Geometry: final body of the model. Coordinates: model frame, mm. Face numbers are marked on the shaded views. A direction names the side the tool comes from. Round coordinates to 2 decimals unless told otherwise and drop trailing zeros. Loops run counter-clockwise (first coordinate to the right, second up) from the corner with the lowest first, then second, coordinate; pieces in that order, holes last. Notation, with made-up numbers: M 52.5,46.25 L 59.5,46.25 A13 cw 59.5,57.25 Z; hole C 59.5,38 d7. An arc over 180 degrees is marked long. Return JSON: item names as keys, results as strings.
from build123d import *

# Parameters (mm, degrees)
PAD003_DEPTH    = 7.5
SKETCH007_W     = 37
SKETCH007_H     = 37
SKETCH007_W_2   = 32.5
SKETCH007_H_2   = 32.5
PAD004_DEPTH    = 66.72
CHAMFER_SIZE    = 2
CHAMFER001_SIZE = 2.9999
POCKET_DEPTH    = 74.421
POCKET001_DEPTH = 18.501


with BuildPart() as part:
    # Sketch006 → Pad003 (new body, symmetric)
    with BuildSketch(Plane.XY):
        Polygon((-16.25, 16.25), (16.25, 16.25), (16.25, -16.25), (6, -16.25), (6, -13.25), (13.25, -13.25), (13.25, 13.25), (-13.25, 13.25), (-13.25, -13.25), (-6, -13.25), (-6, -16.25), (-16.25, -16.25), align=None)
    extrude(amount=PAD003_DEPTH, both=True)

    # Sketch007 (on DatumPlane) → Pad004 (join)
    with BuildSketch(Plane.XY.offset(66.92)):
        Rectangle(SKETCH007_W, SKETCH007_H)
        Rectangle(SKETCH007_W_2, SKETCH007_H_2, mode=Mode.SUBTRACT)
    extrude(amount=-PAD004_DEPTH)

    # Chamfer
    chamfer_edges = [part.edges().sort_by_distance(p)[0] for p in [
        (18.5, -18.5, 33.56),
        (-18.5, -18.5, 33.56),
        (-18.5, 18.5, 33.56),
        (18.5, 18.5, 33.56),
        (-16.25, -16.25, 37.21),
        (16.25, 16.25, 37.21),
        (16.25, -16.25, 37.21),
        (-16.25, 16.25, 37.21),
        (-13.25, 13.25, 0),
        (13.25, 13.25, 0),
        (13.25, -13.25, 0),
        (-13.25, -13.25, 0),
        (16.25, -16.25, -3.65),
        (-16.25, -16.25, -3.65),
        (-16.25, 16.25, -3.65),
        (16.25, 16.25, -3.65),
    ]]
    chamfer(chamfer_edges, length=CHAMFER_SIZE)

    # Chamfer001
    chamfer001_edges = [part.edges().sort_by_distance(p)[0] for p in [
        (-16.25, 0, 7.5),
        (-15.25, 15.25, 7.5),
        (0, 16.25, 7.5),
        (15.25, 15.25, 7.5),
        (16.25, 0, 7.5),
        (15.25, -15.25, 7.5),
        (10.125, -16.25, 7.5),
        (-15.25, -15.25, 7.5),
        (-10.125, -16.25, 7.5),
    ]]
    chamfer(chamfer001_edges, length=CHAMFER001_SIZE)

    # Sketch (on DatumPlane) → Pocket (cut, through all)
    with BuildSketch(Plane.XY.offset(66.92)):
        Polygon((-13.2501, -13.007401), (-13.25, -11.25), (-11.25, -13.25), (-13.007401, -13.2501), align=None)
        Polygon((11.25, -13.25), (13.007401, -13.2501), (13.2501, -13.007401), (13.25, -11.25), align=None)
        Polygon((-13.25, 11.25), (-11.25, 13.25), (-13.007501, 13.25), (-13.2501, 13.007401), align=None)
        Polygon((11.25, 13.25), (13.25, 11.25), (13.2501, 13.007401), (13.007401, 13.2501), align=None)
    extrude(amount=-POCKET_DEPTH, mode=Mode.SUBTRACT)

    # Sketch008 → Pocket001 (cut, through all)
    with BuildSketch(Plane(origin=(0, 0, -17.5), x_dir=(-1, 0, 0), z_dir=(0, -1, 0))):
        with BuildLine():
            Line((-6, -10), (6, -10))
            Line((6, -10), (6, -20))
            ThreePointArc((-6, -20), (0, -26), (6, -20))
            Line((-6, -20), (-6, -10))
        make_face()
    extrude(amount=POCKET001_DEPTH, mode=Mode.SUBTRACT)


solid = part.part
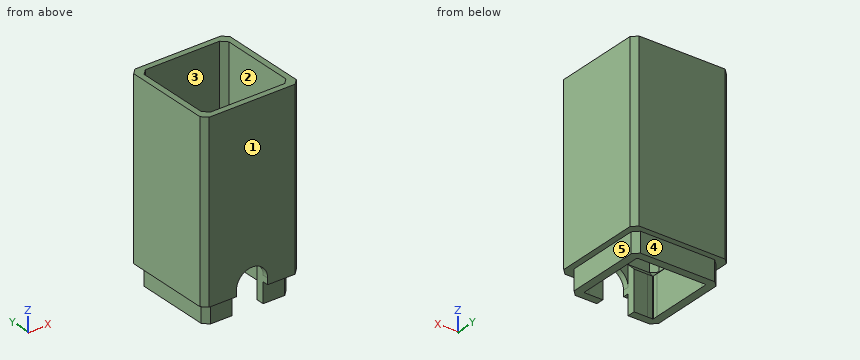
Q1. Pull-direction query (Y, two-part tool) for the marked faces 3, 4 and 5; classes: pulls with the +Y half, pulls with the -Y half, needs draft (parallel to the pull), parting line crosses it, or undercut.
Determined:
{"face 3": "undercut", "face 4": "pulls with the +Y half", "face 5": "needs draft"}
Q2. Material intervals for L1, parallel to Y at x = -9, z = 30; L2, parallel to X at y = -4, z = -1, sorted ascending.
Determined:
{"L1": "y = -18.5 to -16.25, 16.25 to 18.5", "L2": "x = -16.25 to -13.25, 13.25 to 16.25"}
Q3. Pin query (flat end, axial travel): pin 1 (6 mm diameter, centred on x = 8.5, z = -2.5, fed in from -Y); pin 2 (1.4 mm diameter, centred on y = -12, z = -1.5, fed in from -X); pin 3 (1.9 mm diameter, centred on x = 12.5, z = -3.5, fed in from +Y); pin 4 (0.9 mm diameter, centred on x = 12.5, z = -0.5, fed in from -Y). Return the tip coordinate at first contact, or that it passes through.
Determined:
{"pin 1": "stops at y = -18.5", "pin 2": "stops at x = -16.25", "pin 3": "stops at y = 16.25", "pin 4": "stops at y = -16.25"}
Q4. Section query C-C (z = -1.5). Output: boundary loops of the cut face in (x, y), plus the area to 3 significant figures.
Determined:
{"outline": "M -16.25,-14.25 L -14.25,-16.25 L -6,-16.25 L -6,-13.25 L -11.25,-13.25 L -13.01,-13.25 L -13.25,-13.01 L -13.25,-11.25 L -13.25,11.25 L -13.25,13.01 L -13.01,13.25 L 11.25,13.25 L 13.01,13.25 L 13.25,13.01 L 13.25,11.25 L 13.25,-11.25 L 13.25,-13.01 L 13.01,-13.25 L 11.25,-13.25 L 6,-13.25 L 6,-16.25 L 14.25,-16.25 L 16.25,-14.25 L 16.25,14.25 L 14.25,16.25 L -14.25,16.25 L -16.25,14.25 Z", "area": "310 mm^2"}
Q5. Section query B-B (z = 62). Output: boundary loops of the cut face in (x, y), plus the area to 3 significant figures.
Determined:
{"outline": "M -18.5,-16.5 L -16.5,-18.5 L 16.5,-18.5 L 18.5,-16.5 L 18.5,16.5 L 16.5,18.5 L -16.5,18.5 L -18.5,16.5 Z; hole M -16.25,-14.25 L -14.25,-16.25 L 14.25,-16.25 L 16.25,-14.25 L 16.25,14.25 L 14.25,16.25 L -14.25,16.25 L -16.25,14.25 Z", "area": "313 mm^2"}
Q6. Reachability of the marked faces 1 and 2 from +Z, -Z, +X, -X, +Y, -Y: full face, straight path, thin tool, end or side. Return the list, or none.
Determined:
{"face 1": "+Z, -Z, +X, -X, -Y", "face 2": "+Z"}
